```python
from build123d import *

# Parameters (mm, degrees)
SKETCH1_W       = 50
SKETCH1_H       = 50
SKETCH1_R       = 1.5
SUPPORT_DEPTH   = 8
NORTH_START     = -25
SKETCH2_W       = 20
SKETCH2_H       = 5
NORTH_CUT_DEPTH = 4
WEST_START      = -25
SKETCH3_W       = 20
SKETCH3_H       = 5
WEST_CUT_DEPTH  = 4


with BuildPart() as part:
    # Sketch1 → Support (new body)
    with BuildSketch(Plane(origin=(0, 0, 0), x_dir=(1, 0, 0), z_dir=(0, 1, 0))):
        Rectangle(SKETCH1_W, SKETCH1_H)
        with Locations(Location((-21, -21, 0), (0, 0, 270))):
            Circle(SKETCH1_R, mode=Mode.SUBTRACT)
        with Locations(Location((21, -21, 0), (0, 0, 270))):
            Circle(SKETCH1_R, mode=Mode.SUBTRACT)
        with BuildLine():
            Line((-13.031373033, 17.5), (17.5, 17.5))
            Line((17.5, 17.5), (17.5, -17.5))
            Line((17.5, -17.5), (-17.5, -17.5))
            Line((-17.5, -17.5), (-17.5, 13.031373033))
            ThreePointArc((-17.5, 13.031373033), (-20, 14.354248689), (-21, 17))
            Line((-21, 17), (-22.130136986, 20.01369863))
            ThreePointArc((-22.130136986, 20.01369863), (-22.060660172, 22.060660172), (-20.01369863, 22.130136986))
            Line((-20.01369863, 22.130136986), (-17, 21))
            ThreePointArc((-17, 21), (-14.354248689, 20), (-13.031373033, 17.5))
        make_face(mode=Mode.SUBTRACT)
        with Locations(Location((21, 21, 0), (0, 0, 270))):
            Circle(SKETCH1_R, mode=Mode.SUBTRACT)
    extrude(amount=SUPPORT_DEPTH)

    # Sketch2 → North Cut (cut)
    with BuildSketch(Plane.XY.offset(NORTH_START)):
        with Locations((0, 4)):
            Rectangle(SKETCH2_W, SKETCH2_H)
    extrude(amount=NORTH_CUT_DEPTH, mode=Mode.SUBTRACT)

    # Sketch3 → West Cut (cut)
    with BuildSketch(Plane(origin=(0, 0, 0), x_dir=(0, 0, -1), z_dir=(1, 0, 0)).offset(WEST_START)):
        with Locations((0, 4)):
            Rectangle(SKETCH3_W, SKETCH3_H)
    extrude(amount=WEST_CUT_DEPTH, mode=Mode.SUBTRACT)


solid = part.part
```
Work out the finished part from the listing and answer in its coordinate system (mm). A direction names the side the tool comes from. Coordinates: 2 decimals unless noted, no trailing zeros. Write each loop counter-clockwise with the first axis right and the second up, starting at its lowest first coordinate (ties: lowest second). Pieces come first, ordered by that corner, then holes. Notation, with made-up numbers: (-26.5, 60) - (-16.5, 60) arc R35 ccw to (-16.5, 93) - close; hole circle Ø1 at (20.25, 19.5). An arc over 180 degrees is marked (long way). Answer as a JSON object with one key per item and string values.
Q1. Find section D-D (x = 21). Write down the section's boundary in (y, z).
Results list:
{"outline": "(0, -25) - (8, -25) - (8, -22.5) - (0, -22.5) - close; (0, -19.5) - (8, -19.5) - (8, 19.5) - (0, 19.5) - close; (0, 22.5) - (8, 22.5) - (8, 25) - (0, 25) - close"}
Q2. Given pin 1 Ø1.8 at (x, z) = (-21, 21) entering from +Y, flat-ended and moving along its own axis, determine where the tip first touches the part or whether it passes through.
Results list:
{"pin 1": "passes through"}
Q3. Find section B-B (y = 4.5). Write down the section's boundary in (x, z).
Results list:
{"outline": "(-25, -25) - (-10, -25) - (-10, -21) - (10, -21) - (10, -25) - (25, -25) - (25, 25) - (-25, 25) - (-25, 10) - (-21, 10) - (-21, -10) - (-25, -10) - close; hole circle Ø3 at (-21, 21); hole (-22.13, -20.01) arc R1.5 ccw to (-20.01, -22.13) - (-17, -21) arc R4 ccw to (-13.03, -17.5) - (17.5, -17.5) - (17.5, 17.5) - (-17.5, 17.5) - (-17.5, -13.03) arc R4 ccw to (-21, -17) - close; hole circle Ø3 at (21, -21); hole circle Ø3 at (21, 21)"}
Q4. For a pull along Y with two mould halves and no side action, classify faces 1 (the flat face through (-23, 8, 0)), 2 (the flat face through (-10, 4, -23)), 3 (the cylindrical face through (-22.08, 3.94, -22.04)) as pulls with the +Y half, pulls with the -Y half, needs draft (parallel to the pull), parting line crosses it, or undercut.
Results list:
{"face 1": "pulls with the +Y half", "face 2": "undercut", "face 3": "needs draft"}
Q5. Find section A-A (z = 21). Write down the section's boundary in (x, y).
Results list:
{"outline": "(-25, 0) - (-22.5, 0) - (-22.5, 8) - (-25, 8) - close; (-19.5, 0) - (19.5, 0) - (19.5, 8) - (-19.5, 8) - close; (22.5, 0) - (25, 0) - (25, 8) - (22.5, 8) - close"}
Q6. Find section C-C (x = -2.5). Write down the section's boundary in (y, z), plus the area to 3 significant figures.
Results list:
{"outline": "(0, -25) - (1.5, -25) - (1.5, -21) - (6.5, -21) - (6.5, -25) - (8, -25) - (8, -17.5) - (0, -17.5) - close; (0, 17.5) - (8, 17.5) - (8, 25) - (0, 25) - close", "area": "100 mm^2"}
Q7. Which of the six approach directions +Z, -Z, +X, -X, +Y, -Y give full straight-line access (tool end or side, diameter ignored) to faces 4 (the cylindrical face through (-14.385, 3.944, -20.027)), 5 (the flat face through (-23, 6.5, 0)), 6 (the flat face through (0, 6.5, -23))?
Results list:
{"face 4": "+Y, -Y", "face 5": "-X", "face 6": "-Z"}
Q8. Consider L1, parallel to X at y = 2, z = 21; L2, parallel to X at y = 1.25, z = -2.5; L3, parallel to X at y = 2.75, z = 4.5. Determine where each line is inside the solid, lowest interval first. Write a range as from..to.
Results list:
{"L1": "x = -25..-22.5, -19.5..19.5, 22.5..25", "L2": "x = -25..-17.5, 17.5..25", "L3": "x = -21..-17.5, 17.5..25"}
